Autodesk Inventor part; units mm, degrees
ref_plane "YZ Plane" through (0, 0, 0) normal (1, 0, 0) x (0, 1, 0)
ref_plane "XZ Plane" through (0, 0, 0) normal (0, 1, 0) x (-1, 0, 0)
ref_plane "XY Plane" through (0, 0, 0) normal (0, 0, 1) x (1, 0, 0)
sketch "Esquisse1" plane through (0, 0, 0) normal (0, 0, 1) x (1, 0, 0)
  line L0 (-10, 46) -> (10, 46) construction
  line L1 (10, 46) -> (10, -46)
  line L2 (10, -46) -> (-10, -46)
  line L3 (-10, -46) -> (-10, 46)
  line L4 (-10, 46) -> (10, -46) construction
  line L5 (10, 46) -> (-10, -46) construction
  arc A0 (10, 46) -> (-10, 46) centre (0, 46) ccw
  circle A1 centre (0, 46) radius 2.5
  line L6 (0, 46) -> (0, 16.2) construction
  circle A2 centre (0, 16.2) radius 2.5
  point P0 (0, 0)
  dimension "d0" = 29.8
  dimension "d1" = 5
  dimension "d2" = 20
  dimension "d3" = 92
extrude "Extrusion1" add sketch "Esquisse1" along normal blind 5
sketch "Esquisse2" plane through (-10, -46, 0) normal (0, -1, 0) x (1, 0, 0)
  line L0 (-22.4, -56) -> (-22.4, 5)
  line L1 (-22.4, 5) -> (42.4, 5)
  line L2 (42.4, 5) -> (42.4, -56)
  line L3 (42.4, -56) -> (-22.4, -56)
  line L4 (-22.4, -56) -> (42.4, 5) construction
  line L5 (-22.4, 5) -> (42.4, -56) construction
  line L6 (0, 5) -> (20, 5)
  line L7 (0, 5) -> (20, 5)
  line L8 (20, 0) -> (20, 5)
  line L9 (0, 0) -> (0, 5)
  line L10 (0, 0) -> (20, 0)
  line L11 (10, -25.5) -> (10, 0) construction
  line L12 (32.4, -46) -> (-12.4, -46) construction
  line L13 (-12.4, -46) -> (-12.4, -5) construction
  line L14 (-12.4, -5) -> (32.4, -5) construction
  line L15 (32.4, -5) -> (32.4, -46) construction
  line L16 (32.4, -46) -> (-12.4, -5) construction
  line L17 (-12.4, -46) -> (32.4, -5) construction
  circle A0 centre (-12.4, -46) radius 2.1
  circle A1 centre (32.4, -46) radius 2.1
  circle A2 centre (32.4, -5) radius 2.1
  circle A3 centre (-12.4, -5) radius 2.1
  line L18 (-22.4, 5) -> (-29.4, 5)
  line L19 (-29.4, 5) -> (-29.4, -56)
  line L20 (-29.4, -56) -> (-22.4, -56)
  line L21 (-22.4, -56) -> (-22.4, 5)
  line L22 (42.4, 5) -> (49.4, 5)
  line L23 (49.4, 5) -> (49.4, -56)
  line L24 (49.4, -56) -> (42.4, -56)
  line L25 (42.4, -56) -> (42.4, 5)
  dimension "d7" = 64.8
  dimension "d8" = 61
  dimension "d49" = 10
  dimension "d50" = 10
  dimension "d51" = 4.2
  dimension "d53" = 7
extrude "Extrusion2" add sketch "Esquisse2" against normal blind 5
sketch "Esquisse10" plane through (0, 0, 0) normal (0, 0, -1) x (-1, 0, 0)
  line L0 (-4, -10.25) -> (4, -10.25)
  line L1 (4, -10.25) -> (4, -41)
  line L2 (4, -41) -> (-4, -41)
  line L3 (-4, -41) -> (-4, -10.25)
  line L4 (-4, -10.25) -> (4, -41) construction
  line L5 (4, -10.25) -> (-4, -41) construction
  line L6 (0, 0) -> (0, -25.625) construction
  line L7 (-4, -41) -> (4, -41)
  line L8 (4, -41) -> (4, -46)
  line L9 (4, -46) -> (-4, -46)
  line L10 (-4, -46) -> (-4, -41)
  line L11 (-10, -41) -> (10, -41)
  dimension "d41" = 8
  dimension "d48" = 30.75
extrude "Extrusion8" add sketch "Esquisse10" along normal blind 25
extrude "Extrusion10" add sketch "Esquisse2" along normal blind 15 contours L20 L19 L18 L0 | L2 L22 L23 L24
fillet "Congé2" radius 4 2 edges at (35.9, -61, -56) (-35.9, -61, -56)
sketch "Esquisse12" plane through (-39.4, -41, -56) normal (-1, 0, 0) x (0, 0, 1)
  arc A0 (0, -16) -> (4, -20) centre (4, -16) ccw
  line L0 (61, -20) -> (4, -20)
  line L1 (61, 0) -> (61, -20)
  line L2 (0, 0) -> (61, 0)
  line L3 (0, -16) -> (0, 0)
  line L4 (61, -5) -> (0, -5)
  line L5 (0, -5) -> (61, -5)
  line L6 (61, 0) -> (61, -20)
  line L7 (0, -5) -> (61, -5)
  line L8 (61, -5) -> (61, -20)
  line L9 (61, -20) -> (0, -20)
  line L10 (0, -20) -> (0, -5)
  line L11 (0, -5) -> (0, -16)
  line L12 (0, -12.5) -> (15, -12.5) construction
  line L13 (15, -12.5) -> (46, -12.5) construction
  line L14 (46, -12.5) -> (61, -12.5) construction
  circle A1 centre (15, -12.5) radius 2.05
  circle A2 centre (46, -12.5) radius 2.05
  circle A3 centre (15, -12.5) radius 3.75
  circle A4 centre (46, -12.5) radius 3.75
  point P0 (56, 41)
  dimension "d57" = 4.1
  dimension "d59" = 15
  dimension "d62" = 15
  dimension "d63" = 7.5
extrude "Extrusion11" cut sketch "Esquisse12" against normal through all contours A1 | A2
extrude "Extrusion12" cut sketch "Esquisse12" against normal blind 4 contours A3 | A4
sketch "Esquisse13" plane through (39.4, -41, 5) normal (1, 0, 0) x (0, 0, -1)
  circle A0 centre (46, -12.5) radius 3.75
  circle A1 centre (15, -12.5) radius 3.75
  point P0 (5, 41)
extrude "Extrusion13" cut sketch "Esquisse13" against normal blind 4
properties part number "Support_batterie_réduit"
Geometry: final body of the model. Coordinates: model frame, mm. A direction names the side the tool comes from. Coordinates: 2 decimals unless noted, no trailing zeros. Loops run counter-clockwise (first coordinate to the right, second up) from the corner with the lowest first, then second, coordinate; pieces in that order, holes last. Notation, with made-up numbers: M 24.25,31 L 82.25,31 A32 cw 82.25,57 Z; hole C 82.5,59 d3. An arc over 180 degrees is marked long. One line per item, written item: value. Start each with the question number.
1) Cut plane A-A (z = -5). Return loops of the section in (x, y), then the cut area to 3 significant figures.
2) Cut plane B-B (y = 16.2). Return loops of the section in (x, z), then the cut area to 3 significant figures.
3) Draft query along Y for faces 4 (the flat face through (-35.4, -55, -39)), 5 (the flat face through (-36, -61, -23)), 6 (the cylindrical face through (-21.431, -43.535, -47.863)). Return one class per face: released by +Y, released by -Y, zero draft, split by the parting line, or undercut.
4) Material intervals for L1, parallel to X at y = -50, z = -49; L2, parallel to Z at x = -22, y = -43; L3, parallel to Y at x = -34, z = -10, sorted ascending. Write a range as from..to.
5) Pin query (flat end, axial travel): P1, Ø6, axis at x = -7, z = -29, coming from the -Y side; P2, Ø5.5, axis at y = -53.5, z = -10, coming from the -X side; P3, Ø2, axis at y = -55, z = -8.5, coming from the +X side. Return the tip coordinate at first contact, or that it passes through.
6) Cut plane C-C (x = -22.4). Return loops of the section in (y, z).
7) Reachability of faces 1 (the flat face through (-32.4, -53, -26)), 2 (the flat face through (4, -26, -12)), 3 (the flat face through (-10, 2, 2)) from +Z, -Z, +X, -X, +Y, -Y: full face, straight path, thin tool, end or side. Return the list, or none.
8) Cut plane D-D (y = -53.5). Count the separate pieces of the cut face and the enclosed holes in it, then the cut area to 3 significant figures.
Evaluation:
1. outline: M -39.4,-61 L -32.4,-61 L -32.4,-46 L -24.5,-46 L -24.5,-41 L -39.4,-41 Z; M -20.3,-46 L 20.3,-46 L 20.3,-41 L 4,-41 L 4,-10.25 L -4,-10.25 L -4,-41 L -20.3,-41 Z; M 24.5,-46 L 32.4,-46 L 32.4,-61 L 39.4,-61 L 39.4,-41 L 24.5,-41 Z
1. area: 808 mm^2
2. outline: M -10,0 L -2.5,0 L -2.5,5 L -10,5 Z; M 2.5,0 L 10,0 L 10,5 L 2.5,5 Z
2. area: 75.0 mm^2
3. face 4: undercut
3. face 5: released by -Y
3. face 6: zero draft
4. L1: -39.4..-32.4, 32.4..39.4
4. L2: -56..-48.06, -43.94..-7.06, -2.94..5
4. L3: -61..-55.55, -51.45..-41
5. P1: y = -46
5. P2: x = -35.4
5. P3: x = 35.4
6. outline: M -46,-56 L -41,-56 L -41,-48.1 L -46,-48.1 Z; M -46,-43.9 L -41,-43.9 L -41,-7.1 L -46,-7.1 Z; M -46,-2.9 L -41,-2.9 L -41,5 L -46,5 Z
7. face 1: +Z, -Z, -Y
7. face 2: -Z, +X, +Y
7. face 3: +Z, -Z, -X, +Y
8. separate pieces: 6
8. enclosed holes: 0
8. area: 685 mm^2
